from build123d import *

# Parameters (mm, degrees)
SALIENTE_EXTRUIR3_DEPTH = 3
CROQUIS3_R              = 2.5
SALIENTE_EXTRUIR4_DEPTH = 18


with BuildPart() as part:
    # Croquis1 → Saliente-Extruir3 (new body)
    with BuildSketch(Plane.XY):
        Polygon((-54.386636348, 4.299863782), (-50.772905222, 8.802560828), (-52.865489687, 14.183492308), (-58.571805277, 15.061726742), (-62.185536402, 10.559029696), (-60.092951938, 5.178098216), align=None)
    extrude(amount=SALIENTE_EXTRUIR3_DEPTH)

    # Croquis3 → Saliente-Extruir4 (add)
    with BuildSketch(Plane.XY):
        with Locations((-56.479220812, 9.680795262)):
            Circle(CROQUIS3_R)
    extrude(amount=SALIENTE_EXTRUIR4_DEPTH)


solid = part.part
Input: part model. Units: mm. Frame: model coordinates. A direction names the side the tool comes from. Coordinates: 2 decimals unless noted, no trailing zeros. Loops run counter-clockwise (first coordinate to the right, second up) from the corner with the lowest first, then second, coordinate; pieces in that order, holes last. Notation, with made-up numbers: (42, 56.25) - (69, 56.25) arc R28 cw to (69, 76.25) - close; hole circle Ø9 at (2, -3.75). An arc over 180 degrees is marked (long way). Answer in a Markdown table with one row per item. Add a question column.
Item 1: Line query: line 1 along Z through (x, y) = (-55.5, 5); line 2 along Y through (x, z) = (-57, 15); line 3 along Y through (x, z) = (-55, 1.5). Output: solid intervals per line, ascending. Write a range as [from, to].
Item 2: Access query for faces 1 (the flat face through (-58, 7, 3)), 2 (the flat face through (-57.28, 4.745, 1.479)). Directions: +Z, -Z, +X, -X, +Y, -Y. A direction counts if a zero-diameter tool reaches every point of the face in a straight line with its end or side. Return the directions, or none.
Item 3: Contact query for flat-ended pins moving along their axis: P1, Ø1.5, axis at x = -55.5, z = 13, coming from the +Y side; P2, Ø6, axis at y = 8.5, z = 12, coming from the -X side; P3, Ø3, axis at x = -54, z = 8, coming from the -Y side; P4, Ø5, axis at x = -56.5, y = 9, coming from the -Z side. Output: stop coordinate, or through.
Item 4: Section query D-D on x = -53.5. Return the cut outline in (y, z).
Item 5: Section query A-A on z = 2. Return the cut outline in (x, y), then the cut area to 3 significant figures.
Item 6: Section query C-C on y = 7.5. Return the cut outline in (x, z), then the cut area to 3 significant figures.
Item 7: Section query B-B on x = -56.5. Return the cut outline in (y, z), then the cut area to 3 significant figures.
Recorded:
| question | item | result |
|---|---|---|
| 1 | line 1 | [0, 3] |
| 1 | line 2 | [7.24, 12.13] |
| 1 | line 3 | [4.39, 14.51] |
| 2 | face 1 | +Z |
| 2 | face 2 | +Z, -Z, -X, -Y |
| 3 | P1 | y = 12.17 |
| 3 | P2 | x = -58.98 |
| 3 | P3 | y = 7.38 |
| 3 | P4 | z = 0 |
| 4 | outline | (5.4, 0) - (14.28, 0) - (14.28, 3) - (5.4, 3) - close |
| 5 | outline | (-62.19, 10.56) - (-60.09, 5.18) - (-54.39, 4.3) - (-50.77, 8.8) - (-52.87, 14.18) - (-58.57, 15.06) - close |
| 5 | area | 86.6 mm^2 |
| 6 | outline | (-61, 0) - (-51.82, 0) - (-51.82, 3) - (-55.26, 3) - (-55.26, 18) - (-57.7, 18) - (-57.7, 3) - (-61, 3) - close |
| 6 | area | 64.2 mm^2 |
| 7 | outline | (4.63, 0) - (14.74, 0) - (14.74, 3) - (12.18, 3) - (12.18, 18) - (7.18, 18) - (7.18, 3) - (4.63, 3) - close |
| 7 | area | 105 mm^2 |
